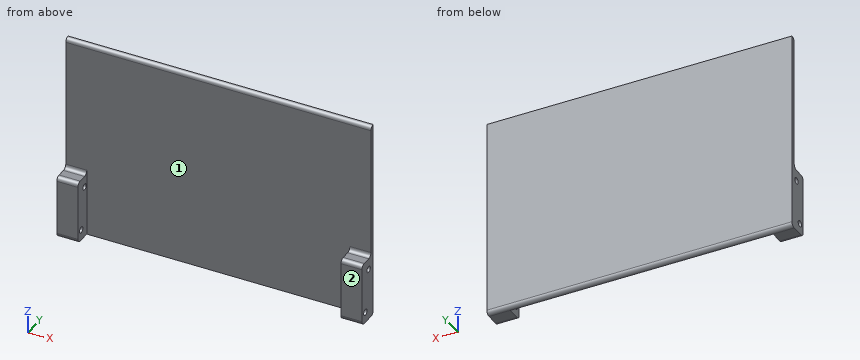
from build123d import *

# Parameters (mm, degrees)
SKETCH_1_W          = 145
SKETCH_1_H          = 95
EXTRUDE_1_DEPTH     = 2
SKETCH_2_W          = 30
SKETCH_2_H          = 8
SKETCH_2_R          = 1.5
EXTRUDE_2_DEPTH     = 145
FILLET_1_R          = 2
CUT_EXTRUDE_2_REACH = 89.25
SKETCH_3_W          = 125
SKETCH_3_H          = 147.268730198


with BuildPart() as part:
    # 草图1 → 凸台-拉伸1 (new body)
    with BuildSketch(Plane(origin=(0, 0, 0), x_dir=(1, 0, 0), z_dir=(0, 1, 0))):
        Rectangle(SKETCH_1_W, SKETCH_1_H)
    extrude(amount=EXTRUDE_1_DEPTH)

    # 草图2 → 凸台-拉伸2 (add, through all)
    with BuildSketch(Plane(origin=(72.5, 0, 0), x_dir=(0, 0, -1), z_dir=(1, 0, 0))):
        with Locations((32.5, -4)):
            Rectangle(SKETCH_2_W, SKETCH_2_H)
        with Locations((22.719682733, -2.043811777)):
            Circle(SKETCH_2_R, mode=Mode.SUBTRACT)
        with Locations((42.5, -5)):
            Circle(SKETCH_2_R, mode=Mode.SUBTRACT)
    extrude(amount=-EXTRUDE_2_DEPTH)

    # 圆角1
    fillet_1_edges = [part.edges().sort_by_distance(p)[0] for p in [
        (0, 2, -47.5),
        (0, -8, -47.5),
        (0, -8, -17.5),
        (0, 0, -17.5),
        (0, 0, 47.5),
    ]]
    fillet(fillet_1_edges, radius=FILLET_1_R - 0.0001)  # a hair under: the kernel refuses the full size

    # 切除-拉伸2: up to this face of the body (flat: up to its plane)
    cut_extrude_2_end = Plane(part.part.faces().sort_by_distance((0, 0, 15))[0])
    # 草图3 → 切除-拉伸2 (cut, up to the picked face)
    with BuildSketch(Plane.XZ.offset(8), mode=Mode.PRIVATE) as cut_extrude_2_sk1:
        Rectangle(SKETCH_3_W, SKETCH_3_H)
    cut_extrude_2_tool1 = split(extrude(cut_extrude_2_sk1.sketch, amount=-CUT_EXTRUDE_2_REACH, mode=Mode.PRIVATE), bisect_by=cut_extrude_2_end, keep=Keep.BOTH, mode=Mode.PRIVATE)
    add(cut_extrude_2_tool1.solids().sort_by(Axis((0, -8, 0), (0, 1, 0)))[0], mode=Mode.SUBTRACT)


solid = part.part
The model under review builds one solid part; all positions refer to its coordinate system, in mm. Face numbers are marked on the shaded views. Give positions to 0.01 mm unless a question says otherwise; leave off trailing zeros. Write each loop counter-clockwise with the first axis right and the second up, starting at its lowest first coordinate (ties: lowest second). Pieces come first, ordered by that corner, then holes.
1. Add section A-A, the plane z = -42.5. Write out the cut boundary in (x, y).
2. Add section C-C, the plane z = 14. Write out the cut boundary in (x, y), plus the area to 3 significant figures.
3. Draft analysis for pull direction X (two halves, no side actions). For the marked faces 1 and 2, state which applies: +X half, -X half, draft (parallel to the pull), parting line (faces both ways), or undercut.
4. Wall thickness on L1, parallel to X at y = -3.5, z = -18.5; L2, parallel to Y at x = 36, z = 32.5; L3, parallel to Y at x = 69, z = -42.5: over which ranges is each line inside the solid? List them lowest first.
5. For P1, Ø5, axis at y = -2.04, z = -22.72, coming from the +X side; P2, Ø6, axis at x = -5.5, z = 28.5, coming from the -Y side; P3, Ø4.5, axis at x = -69, y = -3.5, coming from the +Z side; P4, Ø3, axis at x = 65, y = -3.5, coming from the +Z side, all flat-tipped, find the tip position at first contact; note any pin that passes through.
Worked answers:
1. outline: (-72.5, -8) - (-62.5, -8) - (-62.5, -6.5) - (-72.5, -6.5) - close; (-72.5, -3.5) - (-62.5, -3.5) - (-62.5, 0) - (62.5, 0) - (62.5, -3.5) - (72.5, -3.5) - (72.5, 2) - (-72.5, 2) - close; (62.5, -8) - (72.5, -8) - (72.5, -6.5) - (62.5, -6.5) - close
2. outline: (-72.5, 0) - (72.5, 0) - (72.5, 2) - (-72.5, 2) - close
2. area: 290 mm2
3. face 1: undercut
3. face 2: draft
4. L1: x = -72.5 to -62.5, 62.5 to 72.5
4. L2: y = 0 to 2
4. L3: y = -8 to -6.5, -3.5 to 2
5. P1: stops at x = 72.5
5. P2: stops at y = 0
5. P3: stops at z = -17.35
5. P4: stops at z = -17.5
